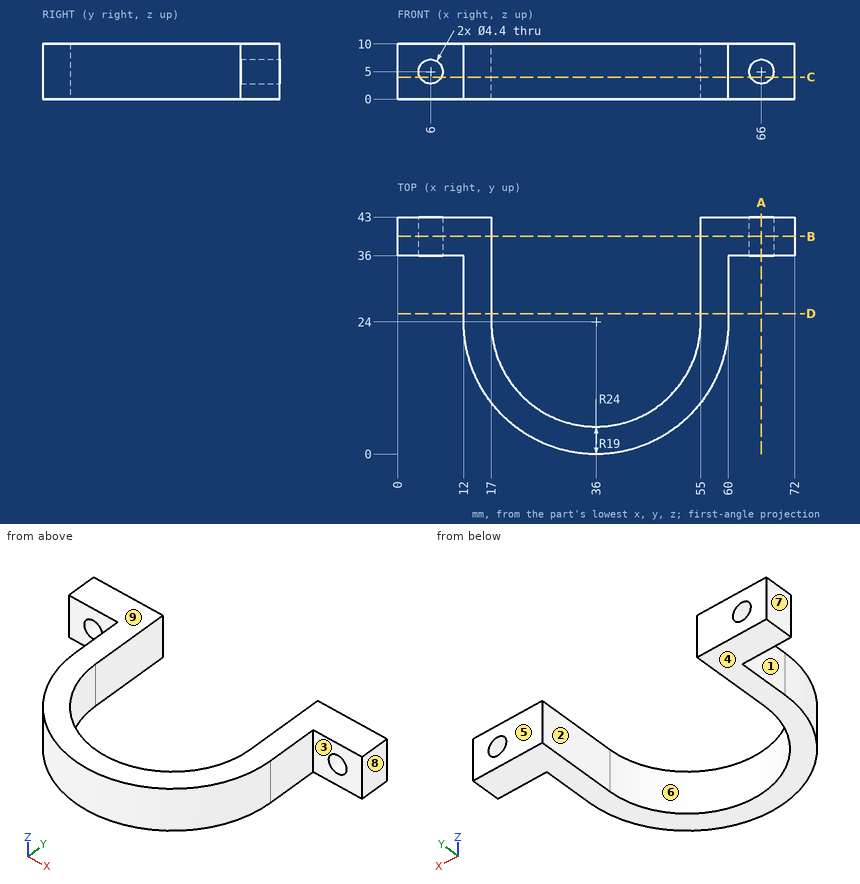
Geometry: see drawing. Coordinates: mm, zero at the bounding-box minimum. A direction names the side the tool comes from. Coordinates: 2 decimals unless noted, no trailing zeros. Loops run counter-clockwise (first coordinate to the right, second up) from the corner with the lowest first, then second, coordinate; pieces in that order, holes last. Notation, with made-up numbers: M -14.5,8.25 L 10.5,8.25 A20 ccw 10.5,46.25 Z; hole C 74.25,17 d3. An arc over 180 degrees is marked long. Put each result on its own line as item: value. Start each with the question number.
1) Reachability of the marked faces 1, 2, 3, 4 and 5 from +Z, -Z, +X, -X, +Y, -Y: full face, straight path, thin tool, end or side. Return the list, or none.
2) Cut plane D-D on y = 25.5. Return the cut outline in (x, z).
3) Cut plane A-A on x = 66. Return the cut outline in (y, z), then the cut area to 3 significant figures.
4) Cut plane C-C on z = 4. Return the cut outline in (x, y).
5) Ray query, L1, parallel to X at y = 40, z = 5; L2, parallel to X at y = 35, z = 4.5; L3, parallel to Z at x = 6, y = 41. Return the intervals inside material, ascending. Write a range as from..to.
6) Cut plane B-B on y = 39.5. Return the cut outline in (x, z), then the cut area to 3 significant figures.
7) Contact query for flat-ended pins moving along their axis: pin 1 Ø1 at (y, z) = (28, 3.5) entering from -X; pin 2 Ø2 at (y, z) = (20, 2) entering from +X; pin 3 Ø3 at (x, z) = (68.5, 6.5) entering from -Y. Output: stop coordinate, or through.
8) Pull-direction query (X, two-part tool) for the marked faces 6, 7, 8 and 9; classes: pulls with the +X half, pulls with the -X half, needs draft (parallel to the pull), parting line crosses it, or undercut.
The answers:
1. face 1: +Z, -Z, -X, -Y
1. face 2: +Z, -Z, +Y
1. face 3: +Z, -Z, +X, -Y
1. face 4: -Z, +X, -X, +Y, -Y
1. face 5: +Z, -Z, +X, -X, +Y
2. outline: M 12,0 L 17,0 L 17,10 L 12,10 Z; M 55,0 L 60,0 L 60,10 L 55,10 Z
3. outline: M 36,0 L 43,0 L 43,2.8 L 36,2.8 Z; M 36,7.2 L 43,7.2 L 43,10 L 36,10 Z
3. area: 39.2 mm²
4. outline: M 0,36 L 4.04,36 L 4.04,43 L 0,43 Z; M 7.96,36 L 12,36 L 12,24 A24 ccw 60,24 L 60,36 L 64.04,36 L 64.04,43 L 55,43 L 55,24 A19 cw 17,24 L 17,43 L 7.96,43 Z; M 67.96,36 L 72,36 L 72,43 L 67.96,43 Z
5. L1: x = 0..3.8, 8.2..17, 55..63.8, 68.2..72
5. L2: x = 12..17, 55..60
5. L3: z = 0..2.8, 7.2..10
6. outline: M 0,0 L 17,0 L 17,10 L 0,10 Z; M 55,0 L 72,0 L 72,10 L 55,10 Z; hole C 6,5 d4.4; hole C 66,5 d4.4
6. area: 310 mm²
7. pin 1: stops at x = 12
7. pin 2: stops at x = 59.81
7. pin 3: stops at y = 36
8. face 6: undercut
8. face 7: pulls with the -X half
8. face 8: pulls with the +X half
8. face 9: needs draft
